```python
from build123d import *

# Parameters (mm, degrees)
SKETCH1_R           = 2.15265
BOSS_EXTRUDE1_DEPTH = 2.54


with BuildPart() as part:
    # Sketch1 → Boss-Extrude1 (new body)
    with BuildSketch(Plane(origin=(0, 0, 0), x_dir=(1, 0, 0), z_dir=(0, 1, 0))):
        with BuildLine():
            Line((178.1875, 29.7875), (-28.1875, 29.7875))
            ThreePointArc((-28.1875, 29.7875), (-30.43256403, 28.85756403), (-31.3625, 26.6125))
            Line((-31.3625, 26.6125), (-31.3625, -21.0125))
            ThreePointArc((-31.3625, -21.0125), (-30.43256403, -23.25756403), (-28.1875, -24.1875))
            Line((-28.1875, -24.1875), (178.1875, -24.1875))
            ThreePointArc((178.1875, -24.1875), (180.43256403, -23.25756403), (181.3625, -21.0125))
            Line((181.3625, -21.0125), (181.3625, 26.6125))
            ThreePointArc((181.3625, 26.6125), (180.43256403, 28.85756403), (178.1875, 29.7875))
        make_face()
        with Locations((-20.25, -13.075)):
            Circle(SKETCH1_R, mode=Mode.SUBTRACT)
        with Locations((75, -13.075)):
            Circle(SKETCH1_R, mode=Mode.SUBTRACT)
        with Locations((170.25, -13.075)):
            Circle(SKETCH1_R, mode=Mode.SUBTRACT)
        Polygon((-1.999996, 7.8), (-1.999996, 9.4), (1.999996, 9.4), (1.999996, 7.8), (7.1, 7.8), (7.1, 5.6), (9.6, 5.6), (9.6, 0), (7.1, 0), (7.1, -2.2), (-7.1, -2.2), (-7.1, 0), (-9.6, 0), (-9.6, 5.6), (-7.1, 5.6), (-7.1, 7.8), align=None, mode=Mode.SUBTRACT)
        Polygon((28.000004, 7.8), (28.000004, 9.4), (31.999996, 9.4), (31.999996, 7.8), (37.1, 7.8), (37.1, 5.6), (39.6, 5.6), (39.6, 0), (37.1, 0), (37.1, -2.2), (22.9, -2.2), (22.9, 0), (20.4, 0), (20.4, 5.6), (22.9, 5.6), (22.9, 7.8), align=None, mode=Mode.SUBTRACT)
        Polygon((58.000004, 7.8), (58.000004, 9.4), (61.999996, 9.4), (61.999996, 7.8), (67.1, 7.8), (67.1, 5.6), (69.6, 5.6), (69.6, 0), (67.1, 0), (67.1, -2.2), (52.9, -2.2), (52.9, 0), (50.4, 0), (50.4, 5.6), (52.9, 5.6), (52.9, 7.8), align=None, mode=Mode.SUBTRACT)
        with Locations((-20.25, 18.675)):
            Circle(SKETCH1_R, mode=Mode.SUBTRACT)
        Polygon((88.000004, 7.8), (88.000004, 9.4), (91.999996, 9.4), (91.999996, 7.8), (97.1, 7.8), (97.1, 5.6), (99.6, 5.6), (99.6, 0), (97.1, 0), (97.1, -2.2), (82.9, -2.2), (82.9, 0), (80.4, 0), (80.4, 5.6), (82.9, 5.6), (82.9, 7.8), align=None, mode=Mode.SUBTRACT)
        Polygon((118.000004, 7.8), (118.000004, 9.4), (121.999996, 9.4), (121.999996, 7.8), (127.1, 7.8), (127.1, 5.6), (129.6, 5.6), (129.6, 0), (127.1, 0), (127.1, -2.2), (112.9, -2.2), (112.9, 0), (110.4, 0), (110.4, 5.6), (112.9, 5.6), (112.9, 7.8), align=None, mode=Mode.SUBTRACT)
        Polygon((148.000004, 7.8), (148.000004, 9.4), (151.999996, 9.4), (151.999996, 7.8), (157.1, 7.8), (157.1, 5.6), (159.6, 5.6), (159.6, 0), (157.1, 0), (157.1, -2.2), (142.9, -2.2), (142.9, 0), (140.4, 0), (140.4, 5.6), (142.9, 5.6), (142.9, 7.8), align=None, mode=Mode.SUBTRACT)
        with Locations((75, 18.675)):
            Circle(SKETCH1_R, mode=Mode.SUBTRACT)
        with Locations((170.25, 18.675)):
            Circle(SKETCH1_R, mode=Mode.SUBTRACT)
    extrude(amount=BOSS_EXTRUDE1_DEPTH)


solid = part.part
```
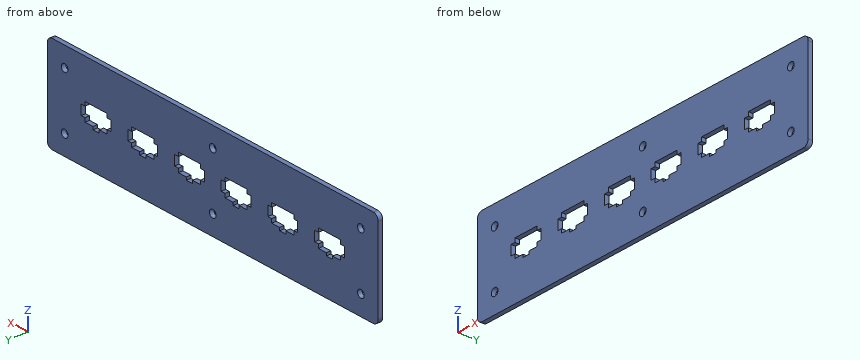
The listing builds one solid part. Answer for the finished solid, in the listing's coordinates (mm). Round coordinates to 2 decimals unless told otherwise and drop trailing zeros. Loops run counter-clockwise (first coordinate to the right, second up) from the corner with the lowest first, then second, coordinate; pieces in that order, holes last.
1) Given P1, Ø5.5, axis at x = -20.25, z = -18.675, coming from the +Y side, flat-ended and moving along its own axis, determine where the tip first touches the part or whether it passes through.
Outcome:
P1: stops at y = 2.54
2) A cutting plane is placed at B-B on y = 2. Give the number of separate pieces and of enclosed holes in the cut face, plus the area to 3 significant figures.
Outcome:
separate pieces: 1
enclosed holes: 12
area: 10,300 mm2
3) A cutting plane is placed at A-A on x = 75. Determine the outline of the cut face in (y, z).
Outcome:
outline: (0, -29.79) - (2.54, -29.79) - (2.54, -20.83) - (0, -20.83) - close; (0, -16.52) - (2.54, -16.52) - (2.54, 10.92) - (0, 10.92) - close; (0, 15.23) - (2.54, 15.23) - (2.54, 24.19) - (0, 24.19) - close
4) Consider line 1 (Z direction, x = 75, y = 1.2); line 2 (X direction, y = 0.8, z = -20); line 3 (Z direction, x = 52.5, y = 2.3). Determine where each line is inside the solid, lowest interval first.
Outcome:
line 1: z = -29.79 to -20.83, -16.52 to 10.92, 15.23 to 24.19
line 2: x = -31.36 to -21.95, -18.55 to 73.3, 76.7 to 168.55, 171.95 to 181.36
line 3: z = -29.79 to -5.6, 0 to 24.19
